The model under review builds one solid part; all positions refer to its coordinate system, in mm. Face numbers are marked on the shaded views. Round coordinates to 2 decimals unless told otherwise and drop trailing zeros. Write each loop counter-clockwise with the first axis right and the second up, starting at its lowest first coordinate (ties: lowest second). Pieces come first, ordered by that corner, then holes. Notation, with made-up numbers: (63.25, 47) - (81.25, 47) arc R28 ccw to (81.25, 81) - close; hole circle Ø8 at (-39.75, -37). An arc over 180 degrees is marked (long way). Write each question's results on one line, items separated by ' | '.
```python
from build123d import *

# Parameters (mm, degrees)
F1_DEPTH = 5
F2_R     = 11.15
F3_DEPTH = 5
F5_COUNT = 3


with BuildPart() as f1:
    # F0 (on Front) → F1 (new body)
    with BuildSketch(Plane.XZ):
        with BuildLine():
            ThreePointArc((12.223679, -10.32384), (15.026291, -5.496414), (16, 0))
            ThreePointArc((16, 0), (-5.648343, 14.969844), (-12.012028, -10.569351))
            ThreePointArc((-12.012028, -10.569351), (-0.562686, -15.990103), (11.239372, -11.38756))
            ThreePointArc((11.239372, -11.38756), (11.711961, -10.837596), (12.223679, -10.32384))
        make_face()
        with BuildLine():
            ThreePointArc((11.239372, -11.38756), (-0.562686, -15.990103), (-12.012028, -10.569351))
            ThreePointArc((-12.012028, -10.569351), (-10.178101, -17.877857), (-12.521378, -25.039323))
            ThreePointArc((-12.521378, -25.039323), (-1.11025, -19.038567), (11.021772, -23.401701))
            ThreePointArc((11.021772, -23.401701), (9.08978, -17.357668), (11.239372, -11.38756))
        make_face()
        with BuildLine():
            ThreePointArc((11.239372, -11.38756), (11.743575, -10.86685), (12.223679, -10.32384))
            ThreePointArc((12.223679, -10.32384), (11.711961, -10.837596), (11.239372, -11.38756))
        make_face()
        with BuildLine():
            ThreePointArc((-13.174834, -25.921247), (-12.839194, -25.486888), (-12.521378, -25.039323))
            ThreePointArc((-12.521378, -25.039323), (-12.855671, -25.47468), (-13.174834, -25.921247))
        make_face()
        with BuildLine():
            ThreePointArc((11.021772, -23.401701), (-1.11025, -19.038567), (-12.521378, -25.039323))
            ThreePointArc((-12.521378, -25.039323), (-12.839194, -25.486888), (-13.174834, -25.921247))
            ThreePointArc((-13.174834, -25.921247), (-15.764732, -37.733723), (-9.348894, -47.984536))
            ThreePointArc((-9.348894, -47.984536), (-9.310283, -48.012249), (-9.271591, -48.039847))
            ThreePointArc((-9.271591, -48.039847), (-4.866336, -50.242007), (0, -51))
            ThreePointArc((0, -51), (7.33666, -49.21877), (13.039785, -44.271678))
            ThreePointArc((13.039785, -44.271678), (15.241991, -39.866387), (16, -35))
            ThreePointArc((16, -35), (15.088679, -29.677241), (12.45853, -24.960825))
            ThreePointArc((12.45853, -24.960825), (11.698135, -24.219982), (11.021772, -23.401701))
        make_face()
        with BuildLine():
            ThreePointArc((12.45853, -24.960825), (11.766004, -24.157439), (11.021772, -23.401701))
            ThreePointArc((11.021772, -23.401701), (11.698135, -24.219982), (12.45853, -24.960825))
        make_face()
        with BuildLine():
            ThreePointArc((0, -51), (-4.866336, -50.242007), (-9.271591, -48.039847))
            ThreePointArc((-9.271591, -48.039847), (-3.003319, -54.882391), (0, -63.662581))
            Line((0, -63.662581), (0, -51))
        make_face()
        with BuildLine():
            Line((13.039785, -47.787126), (13.039785, -44.271678))
            ThreePointArc((13.039785, -44.271678), (7.33666, -49.21877), (0, -51))
            Line((0, -51), (0, -63.662581))
            ThreePointArc((0, -63.662581), (0.011408, -63.756024), (0.022428, -63.849514))
            ThreePointArc((0.022428, -63.849514), (3.912004, -53.695735), (13.039785, -47.787126))
        make_face()
        with BuildLine():
            ThreePointArc((0.022428, -63.849514), (0.011408, -63.756024), (0, -63.662581))
            Line((0, -63.662581), (0, -64.736106))
            ThreePointArc((0, -64.736106), (0.005608, -64.292668), (0.022428, -63.849514))
        make_face()
    extrude(amount=F1_DEPTH)

    # F2 (on Front) → F3 (cut, through all)
    with BuildSketch(Plane.XZ):
        Circle(F2_R)
        with Locations((0, -38.534194)):
            Circle(F2_R)
    extrude(amount=F3_DEPTH, mode=Mode.SUBTRACT)


with BuildPart() as f5_1:
    # F5: instance of F1
    add(f1.part.rotate(Axis((0, 15.020472, 0), (0, 1, 0)), 1 * 360 / F5_COUNT))


with BuildPart() as f5_2:
    # F5: instance of F1
    add(f1.part.rotate(Axis((0, 15.020472, 0), (0, 1, 0)), 2 * 360 / F5_COUNT))


solid = f1.part
```
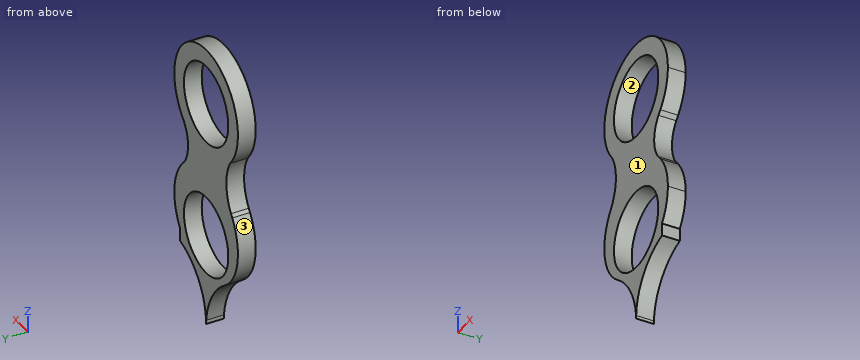
Q1. We need section D-D (x = 14). State the section outline as (y, z) points, plus the area to 3 significant figures.
Evaluation:
outline: (-5, -42.75) - (0, -42.75) - (0, -27.25) - (-5, -27.25) - close; (-5, -7.75) - (0, -7.75) - (0, 7.75) - (-5, 7.75) - close | area: 155 mm^2
Q2. We need section B-B (y = -0.9). State the section outline as (x, z) points, plus the area to 3 significant figures.
Evaluation:
outline: (-13.17, -25.92) arc R16 ccw to (-9.35, -47.98) arc R16.06 ccw to (-9.27, -48.04) arc R22.68 cw to (0, -63.66) - (0, -64.74) arc R17.54 cw to (0.02, -63.85) arc R17.53 cw to (13.04, -47.79) - (13.04, -44.27) arc R16 ccw to (16, -35) arc R16 ccw to (12.46, -24.96) arc R16 ccw to (11.02, -23.4) arc R9.86 cw to (11.24, -11.39) arc R16 ccw to (12.22, -10.32) arc R16 ccw to (16, 0) arc R16 ccw (long way) to (-12.01, -10.57) arc R13.58 cw to (-12.52, -25.04) arc R16 ccw to start; hole circle Ø22.3 at (0, -38.53); hole circle Ø22.3 at (0, 0) | area: 1,010 mm^2
Q3. We need section A-A (x = 2). State the section outline as (y, z) points, plus the area to 3 significant figures.
Evaluation:
outline: (-5, -56.6) - (0, -56.6) - (0, -49.5) - (-5, -49.5) - close; (-5, -27.57) - (0, -27.57) - (0, -10.97) - (-5, -10.97) - close; (-5, 10.97) - (0, 10.97) - (0, 15.87) - (-5, 15.87) - close | area: 143 mm^2
Q4. Insertion check: P1, Ø18, axis at x = 0, z = -38.53, coming from the +Y side; P2, Ø1.8, axis at y = -3, z = -46.5, coming from the +X side; P3, Ø1, axis at x = 3, y = -3, coming from the -Z side; P4, Ø1, axis at y = -2.5, z = -19.5, coming from the -X side. Each pin has a flat end and moves straight along its axis. Give the tip position at first contact, or say it passes through.
Evaluation:
P1: passes through | P2: stops at x = 13.04 | P3: stops at z = -55.71 | P4: stops at x = -10.42
Q5. We need section C-C (z = 5.5). State the section outline as (x, y) points.
Evaluation:
outline: (-15.02, -5) - (-9.7, -5) - (-9.7, 0) - (-15.02, 0) - close; (9.7, -5) - (15.02, -5) - (15.02, 0) - (9.7, 0) - close
Q6. The part is to be moulded in two halves that separate along X. For the marked faces 1, 2 and 3, say which applies: released by +X, released by -X, zero draft, split by the parting line, or undercut.
Evaluation:
face 1: zero draft | face 2: undercut | face 3: released by -X
Q7. For probe 1 along Z at (x, y) = (-3, -2.95); probe 2 along Z at (x, y) = (-2.5, -0.95); probe 3 along X at (y, z) = (-0.8, -10), list the stretches that pass through material, from the lowest coordinate up.
Evaluation:
probe 1: z = -54.89 to -49.27, -27.8 to -10.74, 10.74 to 15.72 | probe 2: z = -55.78 to -49.4, -27.67 to -10.87, 10.87 to 15.8 | probe 3: x = -12.49 to -4.93, 4.93 to 12.49
